Verification items for the finished model (mm, model axes). A direction names the side the tool comes from. Coordinates: 2 decimals unless noted, no trailing zeros. Loops run counter-clockwise (first coordinate to the right, second up) from the corner with the lowest first, then second, coordinate; pieces in that order, holes last. Notation, with made-up numbers: (-16.5, 82) -> (15.5, 82) arc R22 cw to (15.5, 106) -> close; hole circle Ø2 at (-22, -11). An arc over 180 degrees is marked (long way). Write item = value, one per line.
```python
from build123d import *

# Parameters (mm, degrees)
CUT_EXTRUDE2_DEPTH  = 30.863437355
CIRPATTERN1_COUNT   = 13
BOSS_EXTRUDE1_START = -1
BOSS_EXTRUDE1_DEPTH = 1


with BuildPart() as part:
    # Sketch1 → Base-Revolve (revolve)
    with BuildSketch(Plane(origin=(0, 0, 0), x_dir=(0, 0, -1), z_dir=(1, 0, 0)), mode=Mode.PRIVATE) as base_revolve_sk:
        Polygon((0, 12.5), (0, 16.221694663), (-2.228160372, 21), (-3.134468159, 20.577381738), (-1, 16), (-1, 12.5), align=None)
    revolve(base_revolve_sk.sketch.rotate(Axis((0, 0, 14), (0, 0, -1)), 90), axis=Axis((0, 0, 14), (0, 0, -1)))

    # Sketch3 → Cut-Extrude2 (cut, through all)
    with BuildSketch(Plane(origin=(0, 0, 0), x_dir=(-1, 0, 0), z_dir=(0, 0, -1))):
        with BuildLine():
            Line((-2.5, 15.803480629), (-2.5, 20.850659462))
            ThreePointArc((-2.5, 20.850659462), (-5.02562895, 20.389778166), (-7.47614454, 19.62414999))
            Line((-7.47614454, 19.62414999), (-5.130603583, 15.15509508))
            ThreePointArc((-5.130603583, 15.15509508), (-3.829050629, 15.535069079), (-2.5, 15.803480629))
        make_face()
    cut_extrude2 = extrude(amount=-CUT_EXTRUDE2_DEPTH, mode=Mode.SUBTRACT)

    # CirPattern1: Cut-Extrude2 ×13 about axis
    cirpattern1_axis = Axis((0, 0, 0), (0, 0, 1))
    for i in range(1, CIRPATTERN1_COUNT):
        add(cut_extrude2.rotate(cirpattern1_axis, i * 360 / CIRPATTERN1_COUNT), mode=Mode.SUBTRACT)

    # Sketch4 → Boss-Extrude1 (add)
    with BuildSketch(Plane(origin=(0, 0, 0), x_dir=(-1, 0, 0), z_dir=(0, 0, -1)).offset(BOSS_EXTRUDE1_START)):
        with BuildLine():
            Line((-2.5, 12.247448714), (-2.5, 10.5))
            Line((-2.5, 10.5), (2.5, 10.5))
            Line((2.5, 10.5), (2.5, 12.247448714))
            ThreePointArc((2.5, 12.247448714), (0, 12.5), (-2.5, 12.247448714))
        make_face()
    extrude(amount=BOSS_EXTRUDE1_DEPTH)


solid = part.part
```
1) Depth check by flat-ended pin: pin 1 Ø5 at (x, y) = (4, -10) entering from +Z; pin 2 Ø2 at (x, y) = (16.5, -7.5) entering from -Z; pin 3 Ø1 at (x, y) = (-1, -11) entering from +Z; pin 4 Ø16 at (x, y) = (-6.5, -7.5) entering from +Z. Enter the tip coordinate at first touch or a pass-through.
Ans:
pin_1 = 1
pin_2 = 0.42
pin_3 = through
pin_4 = 1.9
2) Material ranges on line 1 (X direction, y = 0, z = 0.2); line 2 (X direction, y = 0, z = 0.4); line 3 (Z direction, x = -14, y = 1.5), recorded low to high.
Ans:
line_1 = -16.65 to -12.5, 12.5 to 16.65
line_2 = -17.08 to -12.5, 12.5 to 17.08
line_3 = 0 to 1
3) Tool access check on faces 1 (the face through (-3.81, 15.54, 0.49)), 2 (the face through (15.88, -1.95, 0.49)), 3 (the face through (12.136, -13.639, 2.052)). Record the directions out of +Z, -Z, +X, -X, +Y, -Y that give a thin tool (end or side, any length) a straight path to the whole face; none if there is none.
Ans:
face_1 = +Z, -Z, +Y
face_2 = +Z, -Z, +X
face_3 = +Z
4) Release check for a two-part mould opening along Y. For faces 4 (the face through (-15.886, -1.91, 0.493)), 5 (the face through (17.086, 11.837, 2.688)), 6 (the face through (5.01, -20.17, 2.69)), 7 (the face through (17.72, 4.67, 1.56)) record: pulls with the +Y half, pulls with the -Y half, needs draft (parallel to the pull), parting line crosses it, or undercut.
Ans:
face_4 = undercut
face_5 = pulls with the +Y half
face_6 = pulls with the -Y half
face_7 = undercut
5) Sectioned sample at B-B, the plane y = 18. Count the separate pieces of the cut face and the enclosed holes in it, plus the area to 3 significant figures.
Ans:
separate_pieces = 3
enclosed_holes = 0
area = 13.8 mm2
6) Sectioned sample at A-A, the plane x = 0. Record the cut outline in (y, z).
Ans:
outline = (-16, 0) -> (-12.5, 0) -> (-12.5, 1) -> (-16, 1) -> close; (10.5, 0) -> (16.22, 0) -> (21, 2.23) -> (20.58, 3.13) -> (16, 1) -> (10.5, 1) -> close
